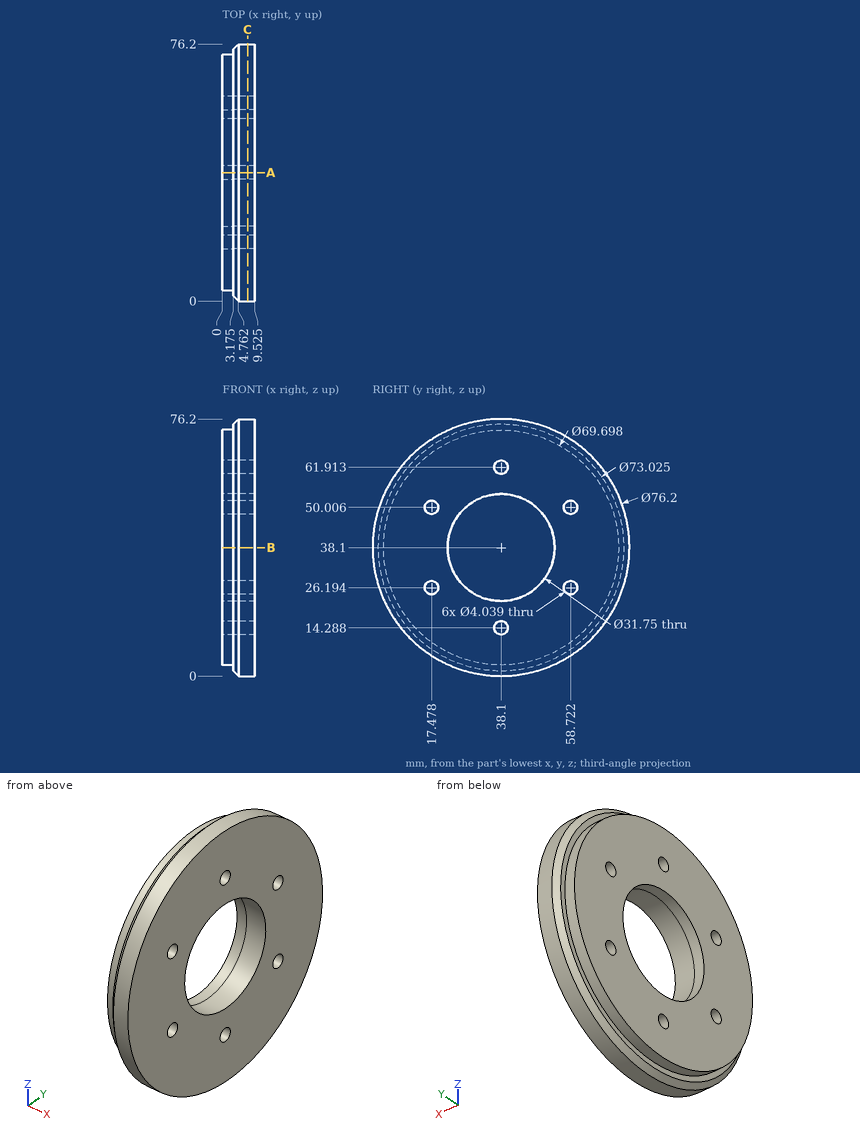
The figure shows three views and two pictorial views of one solid part (mm, origin at its lowest corner). Answer the questions. Give positions to 0.01 mm unless a question says otherwise; leave off trailing zeros. Order: outer loops, then holes, each group sorted by start corner. A loop starts at its lowest first (then second) coordinate and runs counter-clockwise, first axis right, second up. Notation, with made-up numbers: M 22.5,77 L 29.5,77 A23 ccw 29.5,90 Z; hole C 49.5,79.25 d5. An arc over 180 degrees is marked long. Return JSON: item names as keys, results as strings.
1) Each of these flat-tipped pins is pushed along its axis until it touches: pin 1 (2.5 mm diameter, centred on y = 17.48, z = 26.19, fed in from -X); pin 2 (2 mm diameter, centred on x = 5, y = 67, fed in from +Z) (1 decimal); pin 3 (1 mm diameter, centred on x = 5.5, y = 44, fed in from -Z) (1 decimal); pin 4 (4 mm diameter, centred on x = 2.5, z = 43.5, fed in from -Y). Where does it stop, or does it pass through?
Resolved:
{"pin 1": "through", "pin 2": "z = 64", "pin 3": "z = 0.4", "pin 4": "y = 0.63"}
2) Section C-C, the plane x = 7.5 is taken. Give the number of separate pieces and of enclosed holes in the cut face, plus the area to 3 significant figures.
Resolved:
{"separate pieces": "1", "enclosed holes": "7", "area": "3,690 mm^2"}
3) Section B-B, the plane z = 38.1 is taken. Write down the section's boundary in (x, y) (1 decimal), plus the area to 3 significant figures.
Resolved:
{"outline": "M 0,3.3 L 3.2,3.3 L 3.2,1.6 L 4.8,0 L 9.5,0 L 9.5,22.2 L 0,22.2 Z; M 0,54 L 9.5,54 L 9.5,76.2 L 4.8,76.2 L 3.2,74.6 L 3.2,72.9 L 0,72.9 Z", "area": "400 mm^2"}
4) Straight lines are drawn through the part: line 1 along Z through (x, y) = (1.6, 38.1) (1 decimal); line 2 along Z through (x, y) = (6.5, 59.5) (1 decimal); line 3 along Y through (x, z) = (7, 38.1) (1 decimal). For each, find the intervals that lie inside material, in ascending order. Write a range as [from, to].
Resolved:
{"line 1": "[3.3, 12.3], [16.3, 22.2], [54, 59.9], [63.9, 72.9]", "line 2": "[6.6, 24.3], [28.1, 48.1], [51.9, 69.6]", "line 3": "[0, 22.2], [54, 76.2]"}
5) Section A-A, the plane y = 38.1 is taken. Write down the section's boundary in (x, z) (1 decimal).
Resolved:
{"outline": "M 0,3.3 L 3.2,3.3 L 3.2,1.6 L 4.8,0 L 9.5,0 L 9.5,12.3 L 0,12.3 Z; M 0,16.3 L 9.5,16.3 L 9.5,22.2 L 0,22.2 Z; M 0,54 L 9.5,54 L 9.5,59.9 L 0,59.9 Z; M 0,63.9 L 9.5,63.9 L 9.5,76.2 L 4.8,76.2 L 3.2,74.6 L 3.2,72.9 L 0,72.9 Z"}
